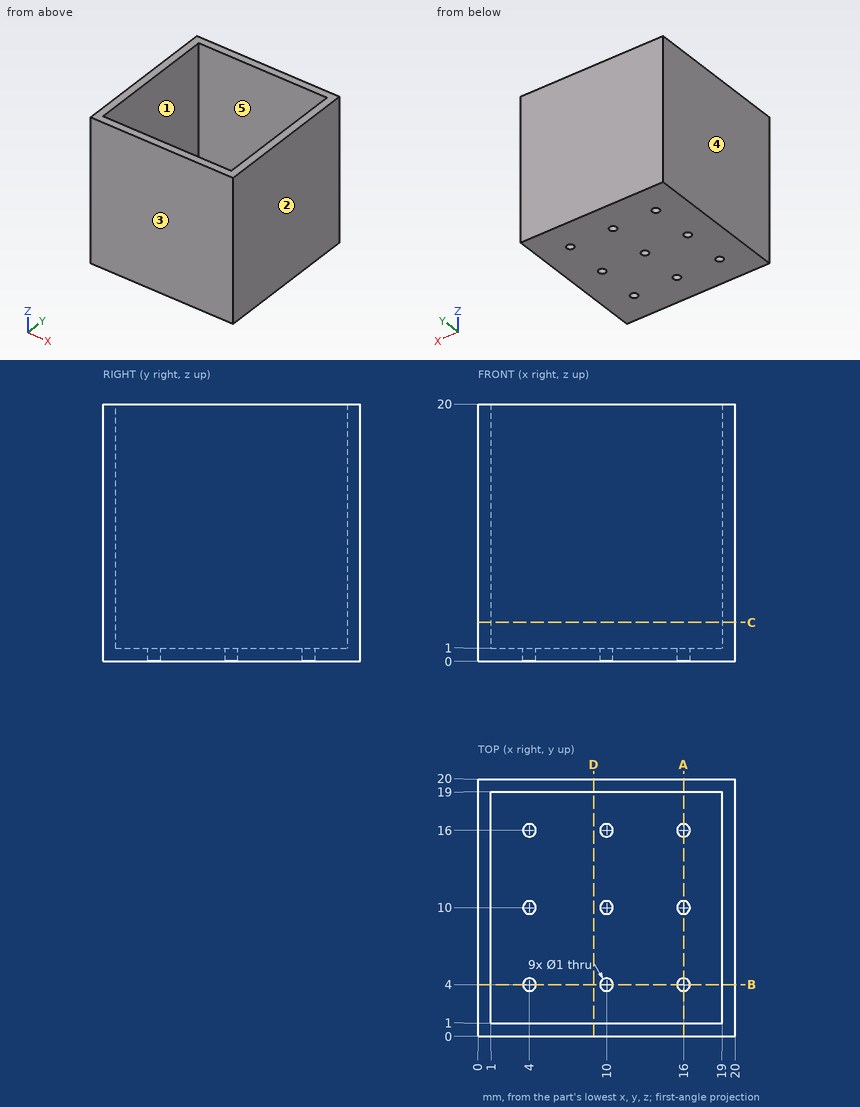
For this review, use the dimensioned drawing (mm, ordinates from the lowest corner) and the shaded views. A direction names the side the tool comes from. Round coordinates to 2 decimals unless told otherwise and drop trailing zeros. Write each loop counter-clockwise with the first axis right and the second up, starting at its lowest first coordinate (ties: lowest second). Pieces come first, ordered by that corner, then holes. Notation, with made-up numbers: (61.25, -3) - (109.25, -3) arc R21 ccw to (109.25, 20) - close; hole circle Ø9 at (-31, 19). An arc over 180 degrees is marked (long way). Answer as a JSON object with one key per item and string values.
1. Tool access review of the marked faces 4 and 5: name each direction out of +Z, -Z, +X, -X, +Y, -Y from which nothing blocks a thin tool from reaching the whole face with its end or side.
Response values:
{"face 4": "+Z, -Z, -X, +Y, -Y", "face 5": "+Z"}
2. To check wall thickness, follow line 1 along Y through (x, z) = (4, 0.75); line 2 along X through (y, z) = (12.25, 18.75). State the ranges of each line that lie inside material, in increasing order.
Response values:
{"line 1": "y = 0 to 3.5, 4.5 to 9.5, 10.5 to 15.5, 16.5 to 20", "line 2": "x = 0 to 1, 19 to 20"}
3. Draft analysis for pull direction X (two halves, no side actions). For the marked faces 1, 2 and 3, state which applies: +X half, -X half, draft (parallel to the pull), parting line (faces both ways), or undercut.
Response values:
{"face 1": "undercut", "face 2": "+X half", "face 3": "draft"}
4. We need section A-A on x = 16. Give the boundary of the cut face in (y, z), then the cut area to 3 significant figures.
Response values:
{"outline": "(0, 0) - (3.5, 0) - (3.5, 1) - (1, 1) - (1, 20) - (0, 20) - close; (4.5, 0) - (9.5, 0) - (9.5, 1) - (4.5, 1) - close; (10.5, 0) - (15.5, 0) - (15.5, 1) - (10.5, 1) - close; (16.5, 0) - (20, 0) - (20, 20) - (19, 20) - (19, 1) - (16.5, 1) - close", "area": "55.0 mm2"}
5. We need section C-C on z = 3. Give the boundary of the cut face in (x, y).
Response values:
{"outline": "(0, 0) - (20, 0) - (20, 20) - (0, 20) - close; hole (1, 1) - (19, 1) - (19, 19) - (1, 19) - close"}
6. We need section D-D on x = 9. Give the boundary of the cut face in (y, z), then the cut area to 3 significant figures.
Response values:
{"outline": "(0, 0) - (20, 0) - (20, 20) - (19, 20) - (19, 1) - (1, 1) - (1, 20) - (0, 20) - close", "area": "58.0 mm2"}
7. For pin 1 Ø6 at (x, y) = (8, 13) entering from +Z, flat-tipped, find the tip position at first contact; note if it passes through.
Response values:
{"pin 1": "stops at z = 1"}
